```python
from build123d import *

# Parameters (mm, degrees)
F0_W     = 40
F0_H     = 20
F1_DEPTH = 40
F2_R     = 6.5
F3_DEPTH = 1.7
F4_R     = 3
F5_DEPTH = 4
F6_R     = 6.5
F7_DEPTH = 1.7
F8_R     = 3
F9_DEPTH = 4


with BuildPart() as f1:
    # F0 (on Top) → F1 (new body)
    with BuildSketch(Plane.XY):
        with Locations((20, 10)):
            Rectangle(F0_W, F0_H)
    extrude(amount=F1_DEPTH)

    # F2 (on face) → F3 (join)
    with BuildSketch(Plane.XY.offset(40)):
        with Locations((9.5, 10)):
            Circle(F2_R)
    extrude(amount=F3_DEPTH)

    # F4 (on face) → F5 (join)
    with BuildSketch(Plane.XY.offset(41.7)):
        with Locations((9.5, 10)):
            Circle(F4_R)
    extrude(amount=F5_DEPTH)

    # F6 (on face) → F7 (join)
    with BuildSketch(Plane(origin=(0, 0, 0), x_dir=(1, 0, 0), z_dir=(0, 0, -1))):
        with Locations((9.5, -10)):
            Circle(F6_R)
    extrude(amount=F7_DEPTH)

    # F8 (on face) → F9 (join)
    with BuildSketch(Plane(origin=(0, 0, -1.7), x_dir=(1, 0, 0), z_dir=(0, 0, -1))):
        with Locations((9.5, -10)):
            Circle(F8_R)
    extrude(amount=F9_DEPTH)


solid = f1.part
```
Geometry: final body of the model. Coordinates: model frame, mm. A direction names the side the tool comes from. Give positions to 0.01 mm unless a question says otherwise; leave off trailing zeros. Write each loop counter-clockwise with the first axis right and the second up, starting at its lowest first coordinate (ties: lowest second). Pieces come first, ordered by that corner, then holes.
1. Section query D-D, the plane x = 26.5. Return loops of the section in (y, z).
2. Section query C-C, the plane y = 15.25. Return loops of the section in (x, z).
3. Section query B-B, the plane y = 10. Return loops of the section in (x, z).
4. Pin query (flat end, axial travel): P1, Ø10, axis at x = 23, y = 10, coming from the +Z side. Return the tip coordinate at first contact, or that it passes through.
5. Line query: probe 1 along Z at (x, y) = (17.5, 2); probe 2 along Z at (x, y) = (12.5, 10.5); probe 3 along Y at (x, z) = (7.5, 41). Output: solid intervals per line, ascending.
6. Reachability of faces 1 (the flat face through (0, 10, 20)), 2 (the cylindrical face through (12, 16, -1)), 3 (the cylindrical face through (12.994, 15.481, 40.838)) from +Z, -Z, +X, -X, +Y, -Y: full face, straight path, thin tool, end or side. Return the list, or none.
7. Section query A-A, the plane x = 9.5. Return loops of the section in (y, z), then the cut area to 3 significant figures.
Computed:
1. outline: (0, 0) - (20, 0) - (20, 40) - (0, 40) - close
2. outline: (0, 0) - (5.67, 0) - (5.67, -1.7) - (13.33, -1.7) - (13.33, 0) - (40, 0) - (40, 40) - (13.33, 40) - (13.33, 41.7) - (5.67, 41.7) - (5.67, 40) - (0, 40) - close
3. outline: (0, 0) - (3, 0) - (3, -1.7) - (6.5, -1.7) - (6.5, -5.7) - (12.5, -5.7) - (12.5, -1.7) - (16, -1.7) - (16, 0) - (40, 0) - (40, 40) - (16, 40) - (16, 41.7) - (12.5, 41.7) - (12.5, 45.7) - (6.5, 45.7) - (6.5, 41.7) - (3, 41.7) - (3, 40) - (0, 40) - close
4. P1: stops at z = 40
5. probe 1: z = 0 to 40
5. probe 2: z = -1.7 to 41.7
5. probe 3: y = 3.82 to 16.18
6. face 1: +Z, -Z, -X, +Y, -Y
6. face 2: -Z
6. face 3: +Z
7. outline: (0, 0) - (3.5, 0) - (3.5, -1.7) - (7, -1.7) - (7, -5.7) - (13, -5.7) - (13, -1.7) - (16.5, -1.7) - (16.5, 0) - (20, 0) - (20, 40) - (16.5, 40) - (16.5, 41.7) - (13, 41.7) - (13, 45.7) - (7, 45.7) - (7, 41.7) - (3.5, 41.7) - (3.5, 40) - (0, 40) - close
7. area: 892 mm2
